Geometry: final body of the model. Coordinates: model frame, mm. A direction names the side the tool comes from. Give positions to 0.01 mm unless a question says otherwise; leave off trailing zeros. Order: outer loops, then holes, each group sorted by start corner. A loop starts at its lowest first (then second) coordinate and runs counter-clockwise, first axis right, second up. Notation, with made-up numbers: (20, -15.75) - (27, -15.75) arc R12 cw to (27, 5.25) - close; hole circle Ø4 at (81.25, -29). An arc over 180 degrees is marked (long way). Put each result on its own line as item: value. Start each with the question number.
1. Ray query, line 1 along X through (y, z) = (39.85, 0); line 2 along Y through (x, z) = (-16.5, -16.5); line 3 along X through (y, z) = (35.8, -15.5). Return the intervals inside material, ascending. Write a range as from..to.
2. Mould query, pull axis Z, two halves, no side actions, for faces 1 (the flat face through (17, 11.125, 17)), 2 (the flat face through (15.958, 9.998, -16.095)), 3 (the flat face through (-18.125, 33.762, 18.202)). Classes: pulls with the +Z half, pulls with the -Z half, needs draft (parallel to the pull), parting line crosses it, or undercut.
3. First-contact query: P1, Ø11, axis at x = 17, z = 14, coming from the +Y side; P2, Ø3.5, axis at y = 55, z = 0, coming from the +X side (3 decimals); P3, Ø2, axis at y = 43, z = -7.5, coming from the -X side; P4, Ø1.2, axis at x = -15, z = -15.5, coming from the +Y side. Flat tips, straight axial feed; report the tip coordinate or a pass-through.
4. Section B-B on z = 0. Return the cut outline in (x, y) (3 decimals), plus the area to 3 significant figures.
5. Section C-C on y = 26. Return the cut outline in (x, z), plus the area to 3 significant figures.
6. Section A-A on y = 10. Return the cut outline in (x, z).
7. Section D-D on x = 6. Return the cut outline in (y, z).
8. Set-up query: faces 4 (the flat face through (-17, 28.753, -17)), 5 (the flat face through (-17, 11.125, 17)), 6 (the flat face through (-16.095, 29.912, -15.958)), 7 (the flat face through (2, 38.329, 2)). Return all of +Z, -Z, +X, -X, +Y, -Y with unobstructed straight access to the full face (end or side cutting, diameter ignored); none if empty.
from build123d import *

# Parameters (mm, degrees)
SKETCH3_W           = 6.441091569
SKETCH3_H           = 9.606110701
CUT_EXTRUDE1_DEPTH  = 22.0218
SKETCH4_W           = 41.8592
SKETCH4_H           = 41.8592
SKETCH4_R           = 18.3896
BOSS_EXTRUDE1_DEPTH = 38.9128
CUT_EXTRUDE2_DEPTH  = 70.806450824
CIRPATTERN1_COUNT   = 4
SKETCH10_R          = 1.25
CUT_EXTRUDE3_DEPTH  = 4


with BuildPart() as part:
    # Sketch2 → Revolve1 (revolve)
    with BuildSketch(Plane.XY, mode=Mode.PRIVATE) as revolve1_sk:
        Polygon((0, 0), (0, 63.2206), (2.5, 63.2206), (2.5, 38.3286), (3.5306, 38.3286), (3.5306, 41.1988), (10.9474, 41.1988), (10.9474, 38.3286), (16.51, 38.3286), (16.51, 38.9128), (20.9296, 38.9128), (20.9296, 0), align=None)
    revolve(revolve1_sk.sketch.rotate(Axis((0, 0, 0), (0, 1, 0)), 90), axis=Axis((0, 0, 0), (0, 1, 0)))

    # Sketch3 → Cut-Extrude1 (cut)
    with BuildSketch(Plane(origin=(0, 63.2206, 0), x_dir=(1, 0, 0), z_dir=(0, 1, 0))):
        with Locations((5.165545785, 1.138296355)):
            Rectangle(SKETCH3_W, SKETCH3_H)
    extrude(amount=-CUT_EXTRUDE1_DEPTH, mode=Mode.SUBTRACT)

    # Sketch4 → Boss-Extrude1 (add)
    with BuildSketch(Plane(origin=(0, 0, 0), x_dir=(1, 0, 0), z_dir=(0, 1, 0))):
        Rectangle(SKETCH4_W, SKETCH4_H)
        Circle(SKETCH4_R, mode=Mode.SUBTRACT)
    extrude(amount=BOSS_EXTRUDE1_DEPTH)

    # Sketch5 → Cut-Extrude2 (cut, symmetric)
    with BuildSketch(Plane(origin=(0, 0, 0), x_dir=(0, 1, 0), z_dir=(0.7071067811865488, 0, 0.7071067811865464))):
        Polygon((0, 25.687324175), (11.1252, 25.687324175), (11.1252, 22.664724175), (8.8392, 22.664724175), (8.8392, 22.410724175), (11.1252, 22.410724175), (28.7528, 22.410724175), (31.0388, 22.410724175), (31.0388, 22.664724175), (28.7528, 22.664724175), (28.7528, 25.687324175), (38.9128, 25.687324175), (48.436079104, 25.687324175), (48.436079104, 38.399610954), (-11.393232354, 38.399610954), (-11.393232354, 25.687324175), align=None)
    cut_extrude2 = extrude(amount=CUT_EXTRUDE2_DEPTH, both=True, mode=Mode.SUBTRACT)

    # CirPattern1: Cut-Extrude2 ×4 about axis
    cirpattern1_axis = Axis((0, 0, 0), (0, 1, 0))
    for i in range(1, CIRPATTERN1_COUNT):
        add(cut_extrude2.rotate(cirpattern1_axis, i * 360 / CIRPATTERN1_COUNT), mode=Mode.SUBTRACT)

    # Sketch10 → Cut-Extrude3 (cut)
    with BuildSketch(Plane(origin=(0, 38.9128, 0), x_dir=(1, 0, 0), z_dir=(0, 1, 0))):
        with Locations(Location((-15.5, 15.5, 0), (0, 0, 270))):
            Circle(SKETCH10_R)
        with Locations(Location((15.5, 15.5, 0), (0, 0, 270))):
            Circle(SKETCH10_R)
        with Locations(Location((15.5, -15.5, 0), (0, 0, 270))):
            Circle(SKETCH10_R)
        with Locations(Location((-15.5, -15.5, 0), (0, 0, 270))):
            Circle(SKETCH10_R)
    extrude(amount=-CUT_EXTRUDE3_DEPTH, mode=Mode.SUBTRACT)


solid = part.part
Resolved:
1. line 1: -10.95..-3.53, -2.5..2.5, 3.53..10.95
1. line 2: 0..11.13, 28.75..38.91
1. line 3: -20.83..-16.75, -14.25..14.25, 16.75..20.83
2. face 1: needs draft
2. face 2: undercut
2. face 3: pulls with the +Z half
3. P1: y = 38.91
3. P2: x = 1.945
3. P3: through
3. P4: y = 34.91
4. outline: (-20.93, 0) - (20.93, 0) - (20.93, 38.913) - (16.51, 38.913) - (16.51, 38.329) - (10.947, 38.329) - (10.947, 41.199) - (3.531, 41.199) - (3.531, 38.329) - (2.5, 38.329) - (2.5, 41.199) - (1.945, 41.199) - (1.945, 63.221) - (-2.5, 63.221) - (-2.5, 38.329) - (-3.531, 38.329) - (-3.531, 41.199) - (-10.947, 41.199) - (-10.947, 38.329) - (-16.51, 38.329) - (-16.51, 38.913) - (-20.93, 38.913) - close
4. area: 1,760 mm^2
5. outline: (-20.93, -10.76) - (-10.76, -20.93) - (10.76, -20.93) - (20.93, -10.76) - (20.93, 10.76) - (10.76, 20.93) - (-10.76, 20.93) - (-20.93, 10.76) - close
5. area: 1,550 mm^2
6. outline: (-20.93, -15.4) - (-15.4, -20.93) - (-11.12, -20.93) - (-20.93, -11.12) - close; (-20.93, -10.76) - (-10.76, -20.93) - (10.76, -20.93) - (20.93, -10.76) - (20.93, 10.76) - (10.76, 20.93) - (-10.76, 20.93) - (-20.93, 10.76) - close; (-20.93, 11.12) - (-11.12, 20.93) - (-15.4, 20.93) - (-20.93, 15.4) - close; (11.12, -20.93) - (15.4, -20.93) - (20.93, -15.4) - (20.93, -11.12) - close; (11.12, 20.93) - (20.93, 11.12) - (20.93, 15.4) - (15.4, 20.93) - close
7. outline: (0, -20.93) - (38.91, -20.93) - (38.91, -15.38) - (38.33, -15.38) - (38.33, -9.16) - (41.2, -9.16) - (41.2, 9.16) - (38.33, 9.16) - (38.33, 15.38) - (38.91, 15.38) - (38.91, 20.93) - (0, 20.93) - close
8. face 4: -Z, -X
8. face 5: +Z, -X
8. face 6: none
8. face 7: +Y
